The listing builds one solid part. Answer for the finished solid, in the listing's coordinates (mm). Face numbers are marked on the shaded views. A direction names the side the tool comes from. Coordinates: 2 decimals unless noted, no trailing zeros. Write each loop counter-clockwise with the first axis right and the second up, starting at its lowest first coordinate (ties: lowest second). Pieces come first, ordered by that corner, then holes. Notation, with made-up numbers: M -14,53 L -6,53 A30 ccw -6,90 Z; hole C -34.75,-10 d11. An arc over 180 degrees is marked long. Answer as CSV lines item,"result". Start each with the question number.
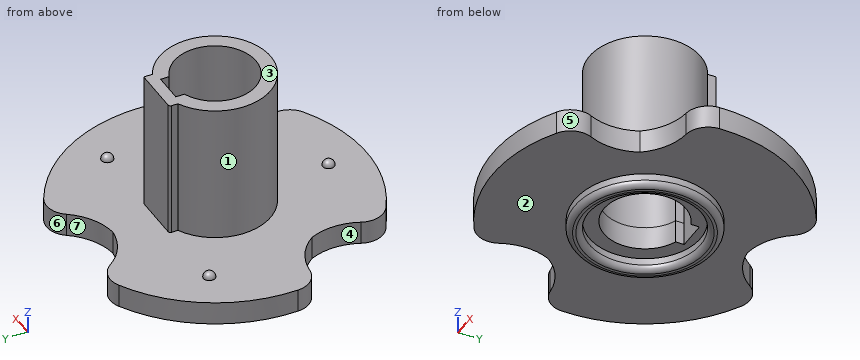
```python
from build123d import *

# Parameters (mm, degrees)
BOSS_EXTRU_1_DEPTH           = 12
ESQUISSE3_R                  = 13
BOSS_EXTRU_5_DEPTH           = 2
BOSS_EXTRU_6_START           = 1.1
ESQUISSE4_R                  = 6
ESQUISSE4_R_2                = 4.75
BOSS_EXTRU_6_DEPTH           = 1.1
ENL_V_MAT_EXTRU_2_REACH      = 23.954
CONG_1_R                     = 0.5
CONG_2_R                     = 0.5
ENL_V_MAT_EXTRU_3_REACH      = 25.108
R_P_TITION_CIRCULAIRE1_COUNT = 2
R_P_TITION_CIRCULAIRE1_ANGLE = 120
R_P_TITION_CIRCULAIRE2_COUNT = 2
R_P_TITION_CIRCULAIRE2_ANGLE = 240
CONG_3_R                     = 0.2
R_P_TITION_CIRCULAIRE3_COUNT = 2
R_P_TITION_CIRCULAIRE3_ANGLE = 240
R_P_TITION_CIRCULAIRE4_COUNT = 2
R_P_TITION_CIRCULAIRE4_ANGLE = 120


with BuildPart() as part:
    # Esquisse1 → Boss.-Extru.1 (new body)
    with BuildSketch(Plane.XY):
        with BuildLine():
            Line((-2.1, 5), (2.1, 5))
            Line((2.1, 5), (2.1, 4.260575079))
            ThreePointArc((2.1, 4.260575079), (0, -4.75), (-2.1, 4.260575079))
            Line((-2.1, 4.260575079), (-2.1, 5))
        make_face()
        with BuildLine():
            Line((-1.25, 4), (1.25, 4))
            Line((1.25, 4), (1.25, 3.269174208))
            ThreePointArc((1.25, 3.269174208), (0, -3.5), (-1.25, 3.269174208))
            Line((-1.25, 3.269174208), (-1.25, 4))
        make_face(mode=Mode.SUBTRACT)
    extrude(amount=BOSS_EXTRU_1_DEPTH)

    # Esquisse3 → Boss.-Extru.5 (add)
    with BuildSketch(Plane(origin=(0, 0, 0), x_dir=(-1, 0, 0), z_dir=(0, 0, -1))):
        Circle(ESQUISSE3_R)
    extrude(amount=BOSS_EXTRU_5_DEPTH)

    # Esquisse4 → Boss.-Extru.6 (add)
    with BuildSketch(Plane(origin=(0, 0, -2), x_dir=(-1, 0, 0), z_dir=(0, 0, -1)).offset(BOSS_EXTRU_6_START)):
        Circle(ESQUISSE4_R)
        Circle(ESQUISSE4_R_2, mode=Mode.SUBTRACT)
    extrude(amount=-BOSS_EXTRU_6_DEPTH)

    # Esquisse5 → Enlèv. mat.-Extru.2 (cut, up to next)
    with BuildSketch(Plane.XY, mode=Mode.PRIVATE) as enl_v_mat_extru_2_sk1:
        with BuildLine():
            Line((1.25, 4), (-1.25, 4))
            Line((-1.25, 4), (-1.25, 3.269174208))
            ThreePointArc((-1.25, 3.269174208), (0, -3.5), (1.25, 3.269174208))
            Line((1.25, 3.269174208), (1.25, 4))
        make_face()
    enl_v_mat_extru_2_tool1 = extrude(enl_v_mat_extru_2_sk1.sketch, amount=-ENL_V_MAT_EXTRU_2_REACH, mode=Mode.PRIVATE) & part.part
    add(enl_v_mat_extru_2_tool1.solids().sort_by_distance((0, 0.133717, 0))[0], mode=Mode.SUBTRACT)

    # Congé1
    cong_1_edges = [part.edges().sort_by_distance(p)[0] for p in [
        (6, 0, -3.1),
    ]]
    fillet(cong_1_edges, radius=CONG_1_R)

    # Congé2
    cong_2_edges = [part.edges().sort_by_distance(p)[0] for p in [
        (4.75, 0, -3.1),
    ]]
    fillet(cong_2_edges, radius=CONG_2_R)

    # Esquisse6 → Enlèv. mat.-Extru.3 (cut, up to next)
    with BuildSketch(Plane(origin=(0, 0, -2), x_dir=(-1, 0, 0), z_dir=(0, 0, -1)), mode=Mode.PRIVATE) as enl_v_mat_extru_3_sk1:
        with BuildLine():
            ThreePointArc((3.60109047, 10.828515139), (2.028708414, 9.38979217), (0, 8.736606683))
            ThreePointArc((0, 8.736606683), (-2.028708414, 9.38979217), (-3.60109047, 10.828515139))
            ThreePointArc((-3.60109047, 10.828515139), (-4.778846502, 11.621991896), (-6.186412192, 11.433647895))
            ThreePointArc((-6.186412192, 11.433647895), (0, 13), (6.186412192, 11.433647895))
            ThreePointArc((6.186412192, 11.433647895), (4.778846502, 11.621991896), (3.60109047, 10.828515139))
        make_face()
    enl_v_mat_extru_3_tool1 = extrude(enl_v_mat_extru_3_sk1.sketch, amount=-ENL_V_MAT_EXTRU_3_REACH, mode=Mode.PRIVATE) & part.part
    enl_v_mat_extru_3 = enl_v_mat_extru_3_tool1.solids().sort_by_distance((0, 11.154072, -2))[0]
    add(enl_v_mat_extru_3, mode=Mode.SUBTRACT)

    # Esquisse7 → Révolution2 (revolve)
    with BuildSketch(Plane.XY):
        with BuildLine():
            Line((-0.495343696, -9.631921937), (0.495343696, -9.768078063))
            ThreePointArc((0.495343696, -9.768078063), (0.068078063, -9.204656304), (-0.495343696, -9.631921937))
        make_face()
    r_volution2 = revolve(axis=Axis((-0.495343696, -9.631921937, 0), (0.9906873922487173, -0.1361561267054709, 0)))

    # Répétition circulaire1: Révolution2 ×2 about axis
    r_p_tition_circulaire1_axis = Axis((0, 0, 0), (0, 0, -1))
    for i in range(1, R_P_TITION_CIRCULAIRE1_COUNT):
        add(r_volution2.rotate(r_p_tition_circulaire1_axis, i * R_P_TITION_CIRCULAIRE1_ANGLE / (R_P_TITION_CIRCULAIRE1_COUNT - 1)))

    # Répétition circulaire2: Révolution2 ×2 about axis
    r_p_tition_circulaire2_axis = Axis((0, 0, 0), (0, 0, -1))
    for i in range(1, R_P_TITION_CIRCULAIRE2_COUNT):
        add(r_volution2.rotate(r_p_tition_circulaire2_axis, i * R_P_TITION_CIRCULAIRE2_ANGLE / (R_P_TITION_CIRCULAIRE2_COUNT - 1)))

    # Congé3
    cong_3_edges = [part.edges().sort_by_distance(p)[0] for p in [
        (-2.1, 5, 6),
    ]]
    fillet(cong_3_edges, radius=CONG_3_R)

    # Répétition circulaire3: Enlèv. mat.-Extru.3 ×2 about axis
    r_p_tition_circulaire3_axis = Axis((0, 0, 0), (0, 0, -1))
    for i in range(1, R_P_TITION_CIRCULAIRE3_COUNT):
        add(enl_v_mat_extru_3.rotate(r_p_tition_circulaire3_axis, i * R_P_TITION_CIRCULAIRE3_ANGLE / (R_P_TITION_CIRCULAIRE3_COUNT - 1)), mode=Mode.SUBTRACT)

    # Répétition circulaire4: Enlèv. mat.-Extru.3 ×2 about axis
    r_p_tition_circulaire4_axis = Axis((0, 0, 0), (0, 0, -1))
    for i in range(1, R_P_TITION_CIRCULAIRE4_COUNT):
        add(enl_v_mat_extru_3.rotate(r_p_tition_circulaire4_axis, i * R_P_TITION_CIRCULAIRE4_ANGLE / (R_P_TITION_CIRCULAIRE4_COUNT - 1)), mode=Mode.SUBTRACT)


solid = part.part
```
1) Each of these flat-tipped pins is pushed along its axis until it touches: P1, Ø2, axis at x = -1.5, z = 6, coming from the +Y side; P2, Ø8, axis at y = -4, z = 7.5, coming from the +X side; P3, Ø3, axis at y = -2, z = 9.5, coming from the -X side; P4, Ø1.5, axis at y = 7.5, z = 2.5, coming from the +X side. Where does it stop, or does it pass through?
2) The part is cut by section C-C (z = -1.5). Determine the outline of the cut face in (x, y), then the cut area to 3 significant figures.
3) Which of the six approach directions +Z, -Z, +X, -X, +Y, -Y give full straight-line access (tool end or side, diameter ignored) to the marked faces 1, 2 and 3?
4) The part is cut by section B-B (y = 0). Determine the outline of the cut face in (x, z), then the cut area to 3 significant figures.
5) For a pull along X with two mould halves and no side action, classify the marked faces 4, 5, 6 and 7 as +X half, -X half, draft (parallel to the pull), parting line (faces both ways), or undercut.
6) The part is cut by section A-A (z = 1.75). Determine the outline of the cut face in (x, y), then the cut area to 3 significant figures.
7) Find the intervals of material crossed by line 1 (Y direction, x = 0, z = 2.75); line 2 (X direction, y = 0, z = 5.25); line 3 (Z direction, x = -7, y = -8), in increasing order. Write a range as from..to.
8) The part is cut by section D-D (y = 9.25). Determine the outline of the cut face in (x, z), then the cut area to 3 significant figures.
Completed:
1,P1,"y = 5"
1,P2,"x = 4.75"
1,P3,"x = -4.72"
1,P4,"through"
2,outline,"M -13,-0.36 A2 ccw -11.18,-2.3 A5 cw -7.57,-4.37 A5 cw -7.58,-8.53 A2 ccw -6.81,-11.07 A13 ccw 6.81,-11.07 A2 ccw 7.58,-8.53 A5 cw 7.57,-4.37 A5 cw 11.18,-2.3 A2 ccw 13,-0.36 A13 ccw 6.19,11.43 A2 ccw 3.6,10.83 A5 cw 0,8.74 A5 cw -3.6,10.83 A2 ccw -6.19,11.43 A13 ccw Z; hole M -1.25,3.27 A3.5 ccw long 1.25,3.27 L 1.25,4 L -1.25,4 Z"
2,area,"409 mm²"
3,face 1,"+Z"
3,face 2,"-Z"
3,face 3,"+Z, +X, -X, +Y, -Y"
4,outline,"M -13,-2 L -6,-2 L -6,-2.6 A0.5 ccw -5.5,-3.1 L -5.25,-3.1 A0.5 ccw -4.75,-2.6 L -4.75,-2 L -3.5,-2 L -3.5,12 L -4.75,12 L -4.75,0 L -13,0 Z; M 3.5,-2 L 4.75,-2 L 4.75,-2.6 A0.5 ccw 5.25,-3.1 L 5.5,-3.1 A0.5 ccw 6,-2.6 L 6,-2 L 13,-2 L 13,0 L 4.75,0 L 4.75,12 L 3.5,12 Z"
4,area,"70.5 mm²"
5,face 4,"-X half"
5,face 5,"+X half"
5,face 6,"undercut"
5,face 7,"undercut"
6,outline,"M -2.1,4.26 A4.75 ccw long 2.1,4.26 L 2.1,5 L -1.9,5 A0.2 ccw -2.1,4.8 Z; hole M -1.25,3.27 A3.5 ccw long 1.25,3.27 L 1.25,4 L -1.25,4 Z"
6,area,"32.7 mm²"
7,line 1,"-4.75..-3.5, 4..5"
7,line 2,"-4.75..-3.5, 3.5..4.75"
7,line 3,"-2..0"
8,outline,"M -9.13,-2 L -1.77,-2 L -1.77,0 L -9.13,0 Z; M 1.77,-2 L 9.13,-2 L 9.13,0 L 1.77,0 Z"
8,area,"29.5 mm²"
